For this review, take the finished solid that the model builds, in its own axes (mm). Coordinates: 2 decimals unless noted, no trailing zeros. Loops run counter-clockwise (first coordinate to the right, second up) from the corner with the lowest first, then second, coordinate; pieces in that order, holes last. Notation, with made-up numbers: (1.25, 77.25) - (48.25, 77.25) arc R20 ccw to (48.25, 101.25) - close; hole circle Ø6 at (8, -15.75). An arc over 180 degrees is marked (long way). One line per item, written item: value. Start each with the question number.
1. Take a section at B-B, the plane y = 480. State the section outline as (x, z) points.
2. Take a section at A-A, the plane z = 0. State the section outline as (x, y) points, and give its area (4 significant figures).
3. To check wall thickness, follow line 1 (Y direction, x = -2, z = 0); line 2 (Z direction, x = -6.25, y = 480); line 3 (Y direction, x = 0.5, z = 1). State the ranges of each line that lie inside material, in increasing order. Write a range as from..to.
```python
from build123d import *

# Parameters (mm, degrees)
SKETCH1_W                = 25
SKETCH1_H                = 25
BOSS_EXTRUDE1_DEPTH      = 500
BOSS_EXTRUDE1_DEPTH_BACK = 100
SKETCH2_R                = 5
CUT_EXTRUDE1_DEPTH       = 500


with BuildPart() as part:
    # Sketch1 → Boss-Extrude1 (new body, two sides)
    with BuildSketch(Plane(origin=(0, 0, 0), x_dir=(1, 0, 0), z_dir=(0, 1, 0))) as boss_extrude1_sk:
        Rectangle(SKETCH1_W, SKETCH1_H)
    extrude(amount=BOSS_EXTRUDE1_DEPTH)
    extrude(boss_extrude1_sk.sketch, amount=-BOSS_EXTRUDE1_DEPTH_BACK)

    # Sketch2 → Cut-Extrude1 (cut)
    with BuildSketch(Plane.ZY.offset(12.5)):
        with Locations((0, 480)):
            Circle(SKETCH2_R)
    extrude(amount=-CUT_EXTRUDE1_DEPTH, mode=Mode.SUBTRACT)


solid = part.part
```
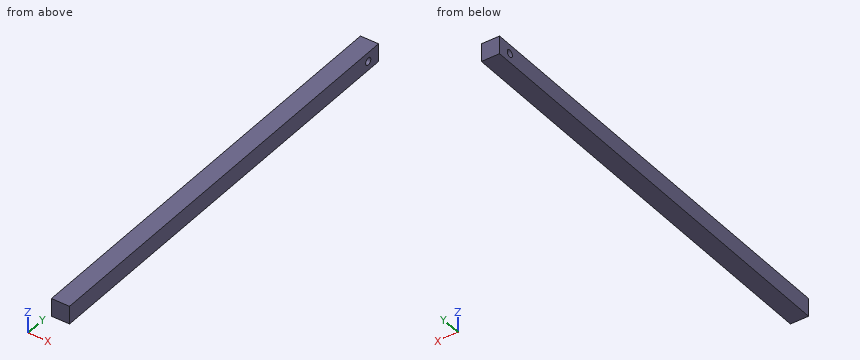
Solutions:
1. outline: (-12.5, -12.5) - (12.5, -12.5) - (12.5, -5) - (-12.5, -5) - close; (-12.5, 5) - (12.5, 5) - (12.5, 12.5) - (-12.5, 12.5) - close
2. outline: (-12.5, -100) - (12.5, -100) - (12.5, 475) - (-12.5, 475) - close; (-12.5, 485) - (12.5, 485) - (12.5, 500) - (-12.5, 500) - close
2. area: 14,750 mm2
3. line 1: -100..475, 485..500
3. line 2: -12.5..-5, 5..12.5
3. line 3: -100..475.1, 484.9..500
